from build123d import *

# Parameters (mm, degrees)
SKETCH_R     = 12
SKETCH_R_2   = 10
PAD_DEPTH    = 2
SKETCH001_R  = 3
PAD001_DEPTH = 2


with BuildPart() as part:
    # Sketch → Pad (new body)
    with BuildSketch(Plane.XY):
        Circle(SKETCH_R)
        Circle(SKETCH_R_2, mode=Mode.SUBTRACT)
    extrude(amount=-PAD_DEPTH)

    # Sketch001 → Pad001 (join)
    with BuildSketch(Plane.XY):
        with Locations((-9.192388, 9.192388)):
            Circle(SKETCH001_R)
        with Locations((9.192388, 9.192388)):
            Circle(SKETCH001_R)
    extrude(amount=-PAD001_DEPTH)


solid = part.part
Work out the finished part from the listing and answer in its coordinate system (mm). Coordinates: 2 decimals unless noted, no trailing zeros. Loops run counter-clockwise (first coordinate to the right, second up) from the corner with the lowest first, then second, coordinate; pieces in that order, holes last. Notation, with made-up numbers: (2, 88.25) -> (26, 88.25) arc R21 cw to (26, 104.25) -> close; hole circle Ø7 at (-40, 6.5). An arc over 180 degrees is marked (long way). Answer as CSV lines item,"result".
1) The part is cut by section C-C (z = -1.4). Give the vertices of the cut face in (x, y), and give its area (3 significant figures).
A:
outline,"(-10.18, 6.36) arc R12 ccw (long way) to (10.18, 6.36) arc R3 ccw (long way) to (6.36, 10.18) arc R12 ccw to (-6.36, 10.18) arc R3 ccw (long way) to start; hole circle Ø20 at (0, 0)"
area,"179 mm²"
2) The part is cut by section A-A (x = 0). Give the vertices of the cut face in (y, z), and give its area (3 significant figures).
A:
outline,"(-12, -2) -> (-10, -2) -> (-10, 0) -> (-12, 0) -> close; (10, -2) -> (12, -2) -> (12, 0) -> (10, 0) -> close"
area,"8.00 mm²"
3) Straight lines are drawn through the part: probe 1 along X at (y, z) = (0, -0.8); probe 2 along X at (y, z) = (-2.25, -1.45); probe 3 along Y at (x, z) = (6, -0.9). For each, find the intervals that lie inside material, in ascending order.
A:
probe 1,"x = -12 to -10, 10 to 12"
probe 2,"x = -11.79 to -9.74, 9.74 to 11.79"
probe 3,"y = -10.39 to -8, 8 to 10.39"
4) For a pull along Y with two mould halves and no side action, classify faces 1 (the face through (-2.17, -9.76, -0.99)), 2 (the face through (4.5, 9.1, -2)), 3 (the face through (0, -12, -1)) as released by +Y, released by -Y, zero draft, split by the parting line, or undercut.
A:
face 1,"undercut"
face 2,"zero draft"
face 3,"undercut"
